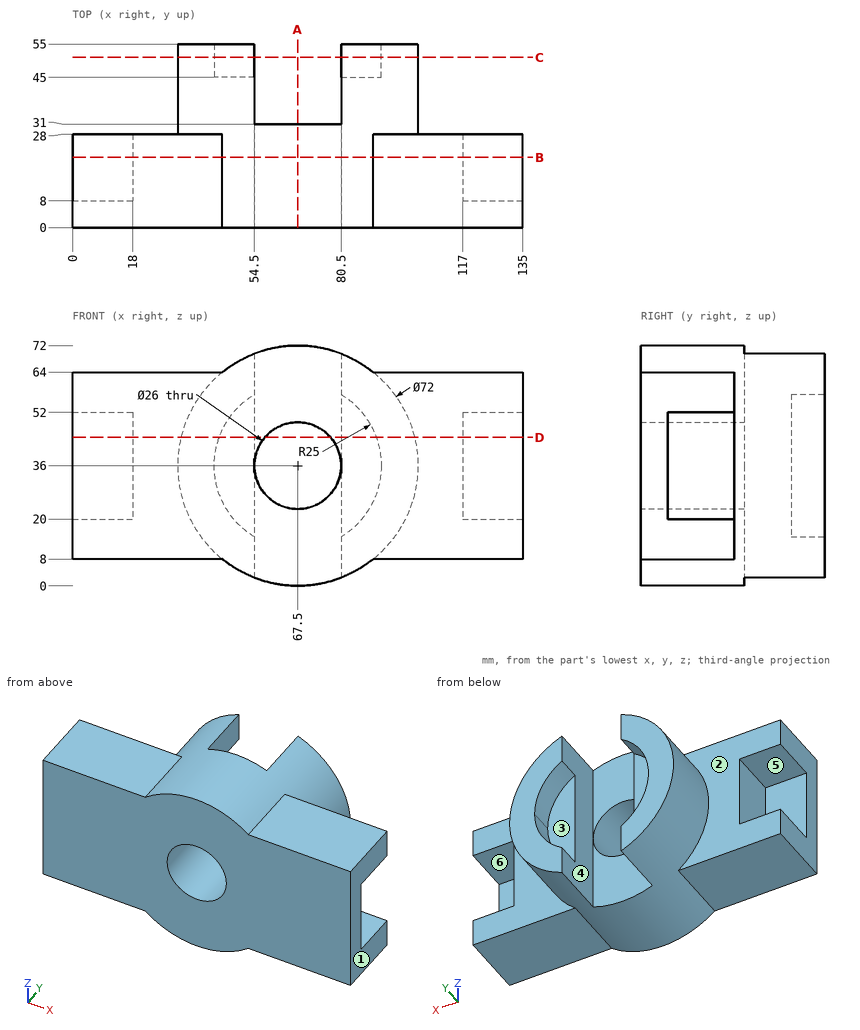
Geometry check sheet. Reference: drawing and pictorial views, mm from the part's lowest x, y, z. A direction names the side the tool comes from. Give positions to 0.01 mm unless a question says otherwise; leave off trailing zeros. Write each loop counter-clockwise with the first axis right and the second up, starting at its lowest first coordinate (ties: lowest second). Pieces come first, ordered by that corner, then holes.
Item 1: Cross-section at D-D (z = 44.5). Enter the section's corners in (x, y), and give its area (3 significant figures).
Item 2: Scan lines: L1, parallel to Z at x = 67, y = 14; L2, parallel to X at y = 24, z = 36; L3, parallel to X at y = 7.5, z = 36. Record each from-to range of solid material in increasing order.
Item 3: Cross-section at A-A (x = 67.5). Enter the section's corners in (y, z), and give its area (3 significant figures).
Item 4: Cross-section at B-B (y = 21). Enter the section's corners in (x, z), and give its area (3 significant figures).
Item 5: Gauge pin test, flat ends, axial feed: pin 1 (5 mm diameter, centred on x = 30.5, y = 23.5, fed in from +Z); pin 2 (10 mm diameter, centred on x = 89, z = 38, fed in from -Y); pin 3 (3 mm diameter, centred on x = 25, z = 56, fed in from +Y); pin 4 (10 mm diameter, centred on x = 103, y = 43.5, fed in from -Z). Record the tip position at first contact, or that the pin passes through.
Item 6: Cross-section at C-C (y = 51). Enter the section's corners in (x, z), and give its area (3 significant figures).
Item 7: Draft check along X on the marked faces 1, 2 and 3. Enter one of: released by +X, released by -X, zero draft, split by the parting line, or undercut.
Item 8: Access from +Z, -Z, +X, -X, +Y, -Y to the whole of each face (thin tool, end or side, straight path). Record for the marked faces 4, 5 and 6.
Report:
1. outline: (0, 0) - (57.66, 0) - (57.66, 31) - (54.5, 31) - (54.5, 45) - (43.99, 45) - (43.99, 55) - (32.52, 55) - (32.52, 28) - (18, 28) - (18, 8) - (0, 8) - close; (77.34, 0) - (135, 0) - (135, 8) - (117, 8) - (117, 28) - (102.48, 28) - (102.48, 55) - (91.01, 55) - (91.01, 45) - (80.5, 45) - (80.5, 31) - (77.34, 31) - close
1. area: 3,500 mm2
2. L1: z = 0 to 23.01, 48.99 to 72
2. L2: x = 18 to 54.5, 80.5 to 117
2. L3: x = 0 to 54.5, 80.5 to 135
3. outline: (0, 0) - (31, 0) - (31, 23) - (0, 23) - close; (0, 49) - (31, 49) - (31, 72) - (0, 72) - close
3. area: 1,430 mm2
4. outline: (0, 8) - (44.87, 8) arc R36 ccw to (90.13, 8) - (135, 8) - (135, 20) - (117, 20) - (117, 52) - (135, 52) - (135, 64) - (90.13, 64) arc R36 ccw to (44.87, 64) - (0, 64) - (0, 52) - (18, 52) - (18, 20) - (0, 20) - close; hole circle Ø26 at (67.5, 36)
4. area: 6,370 mm2
5. pin 1: stops at z = 64
5. pin 2: stops at y = 0
5. pin 3: stops at y = 28
5. pin 4: stops at z = 16.88
6. outline: (54.5, 2.43) - (54.5, 14.65) arc R25 cw to (54.5, 57.35) - (54.5, 69.57) arc R36 ccw to start; (80.5, 2.43) arc R36 ccw to (80.5, 69.57) - (80.5, 57.35) arc R25 cw to (80.5, 14.65) - close
6. area: 1,520 mm2
7. face 1: released by +X
7. face 2: zero draft
7. face 3: undercut
8. face 4: +Z, -Z, +Y
8. face 5: -X, +Y
8. face 6: +X, +Y
